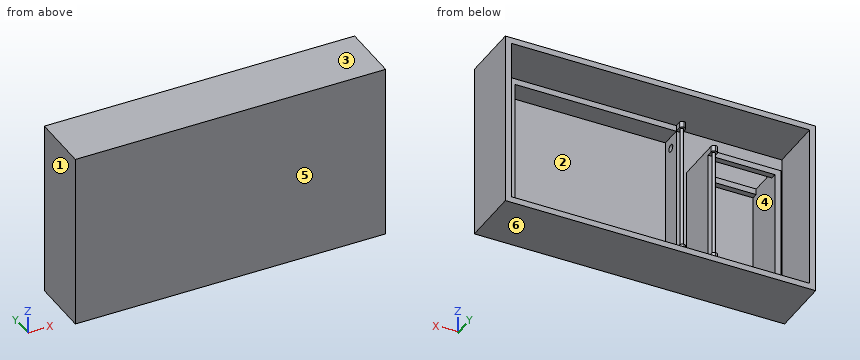
```python
from build123d import *

# Parameters (mm, degrees)
SKETCH1_W              = 127
SKETCH1_H              = 69.85
BASE_DEPTH             = 2.54
SKETCH2_W              = 73.66
SKETCH2_H              = 58.42
SKETCH2_W_2            = 68.58
SKETCH2_H_2            = 53.34
PCB_HOLDER_DEPTH       = 8.89
SKETCH1_3_W            = 132.08
SKETCH1_3_H            = 74.93
SKETCH1_3_W_2          = 127
SKETCH1_3_H_2          = 69.85
BOSS_EXTRUDE5_DEPTH    = 25.4
BOSS_EXTRUDE6_DEPTH    = 17.78
SKETCH7_W              = 25.908
SKETCH7_H              = 12.7
BATTERY_GAP_DEPTH      = 2.54
SKETCH4_R              = 1.5875
WIRE_GAP_DEPTH         = 2.54
SKETCH8_W              = 2.54
SKETCH8_H              = 2.54
PCB_HOLDER_HINGE_DEPTH = 3.81
FILLET4_R              = 1.27
SKETCH13_R             = 0.635
BOSS_EXTRUDE10_DEPTH   = 53.34
SKETCH14_W             = 2.54
SKETCH14_H             = 2.54
BOSS_EXTRUDE11_DEPTH   = 3.81
FILLET5_R              = 1.27
SKETCH15_R             = 0.635
BOSS_EXTRUDE13_DEPTH   = 46.228


with BuildPart() as part:
    # Sketch1 → Base (new body)
    with BuildSketch(Plane(origin=(0, 0, 0), x_dir=(1, 0, 0), z_dir=(0, 1, 0))):
        Rectangle(SKETCH1_W, SKETCH1_H)
    extrude(amount=BASE_DEPTH)

    # Sketch2 → PCB-Holder (add)
    with BuildSketch(Plane(origin=(0, 2.54, 0), x_dir=(1, 0, 0), z_dir=(0, 1, 0))):
        with Locations((20.32, -0.635)):
            Rectangle(SKETCH2_W, SKETCH2_H)
        with Locations((20.32, -0.635)):
            Rectangle(SKETCH2_W_2, SKETCH2_H_2, mode=Mode.SUBTRACT)
    extrude(amount=PCB_HOLDER_DEPTH)

    # Sketch1<3> → Boss-Extrude5 (add)
    with BuildSketch(Plane(origin=(0, 0, 0), x_dir=(1, 0, 0), z_dir=(0, 1, 0))):
        Rectangle(SKETCH1_3_W, SKETCH1_3_H)
        Rectangle(SKETCH1_3_W_2, SKETCH1_3_H_2, mode=Mode.SUBTRACT)
    extrude(amount=BOSS_EXTRUDE5_DEPTH)

    # Sketch6 → Boss-Extrude6 (add)
    with BuildSketch(Plane(origin=(0, 2.54, 0), x_dir=(1, 0, 0), z_dir=(0, 1, 0))):
        Polygon((-51.308, -13.843), (-51.308, 34.925), (-53.848, 34.925), (-53.848, -16.383), (-22.86, -16.383), (-22.86, 34.925), (-25.4, 34.925), (-25.4, -13.843), align=None)
    extrude(amount=BOSS_EXTRUDE6_DEPTH)

    # Sketch7 → Battery-Gap (cut)
    with BuildSketch(Plane.XY.offset(16.383)):
        with Locations((-38.354, 11.43)):
            Rectangle(SKETCH7_W, SKETCH7_H)
    extrude(amount=-BATTERY_GAP_DEPTH, mode=Mode.SUBTRACT)

    # Sketch4 → Wire-Gap (cut)
    with BuildSketch(Plane.ZY.offset(16.51)):
        with Locations((22.225, 6.985)):
            Circle(SKETCH4_R)
    extrude(amount=-WIRE_GAP_DEPTH, mode=Mode.SUBTRACT)

    # Sketch8 → PCB-Holder-Hinge (add)
    with BuildSketch(Plane(origin=(0, 11.43, 0), x_dir=(1, 0, 0), z_dir=(0, 1, 0))):
        with Locations((-15.24, -28.575)):
            Rectangle(SKETCH8_W, SKETCH8_H)
        with Locations((-15.24, 27.305)):
            Rectangle(SKETCH8_W, SKETCH8_H)
    extrude(amount=PCB_HOLDER_HINGE_DEPTH)

    # Fillet4
    fillet4_edges = [part.edges().sort_by_distance(p)[0] for p in [
        (-16.51, 15.24, -27.305),
        (-13.97, 15.24, -27.305),
        (-13.97, 15.24, 28.575),
        (-16.51, 15.24, 28.575),
    ]]
    fillet(fillet4_edges, radius=FILLET4_R - 0.0001)  # a hair under: the kernel refuses the full size

    # Sketch13 → Boss-Extrude10 (add)
    with BuildSketch(Plane.XY.offset(-26.035)):
        with Locations(Location((-15.24, 13.589, 0), (0, 0, 180))):
            Circle(SKETCH13_R)
    extrude(amount=BOSS_EXTRUDE10_DEPTH)

    # Sketch14 → Boss-Extrude11 (add)
    with BuildSketch(Plane(origin=(0, 20.32, 0), x_dir=(1, 0, 0), z_dir=(0, 1, 0))):
        with Locations((-24.13, -15.113)):
            Rectangle(SKETCH14_W, SKETCH14_H)
        with Locations((-24.13, 33.655)):
            Rectangle(SKETCH14_W, SKETCH14_H)
    extrude(amount=BOSS_EXTRUDE11_DEPTH)

    # Fillet5
    fillet5_edges = [part.edges().sort_by_distance(p)[0] for p in [
        (-22.86, 24.13, -33.655),
        (-25.4, 24.13, -33.655),
        (-25.4, 24.13, 15.113),
        (-22.86, 24.13, 15.113),
    ]]
    fillet(fillet5_edges, radius=FILLET5_R - 0.0001)  # a hair under: the kernel refuses the full size

    # Sketch15 → Boss-Extrude13 (add)
    with BuildSketch(Plane.XY.offset(-32.385)):
        with Locations(Location((-24.13, 22.479, 0), (0, 0, 180))):
            Circle(SKETCH15_R)
    extrude(amount=BOSS_EXTRUDE13_DEPTH)


solid = part.part
```
Check sheet for the modelled part. Datum: model origin and axes. Units: mm. Face numbers are marked on the shaded views. A direction names the side the tool comes from. Coordinates: 2 decimals unless noted, no trailing zeros. Loops run counter-clockwise (first coordinate to the right, second up) from the corner with the lowest first, then second, coordinate; pieces in that order, holes last. Notation, with made-up numbers: M -19,56.25 L -5,56.25 A29 cw -5,78.25 Z; hole C -5,9.5 d6. An arc over 180 degrees is marked long. Answer as a JSON object with one key per item and string values.
1. Access from +Z, -Z, +X, -X, +Y, -Y to the whole of each face (thin tool, end or side, straight path). Record for the marked faces 1 and 2.
Outcome:
{"face 1": "+Z, -Z, -X, +Y, -Y", "face 2": "+Y"}
2. Release check for a two-part mould opening along Z. For the marked faces 3, 4, 5 and 6 record: pulls with the +Z half, pulls with the -Z half, needs draft (parallel to the pull), parting line crosses it, or undercut.
Outcome:
{"face 3": "pulls with the +Z half", "face 4": "undercut", "face 5": "needs draft", "face 6": "pulls with the -Z half"}
3. Sectioned sample at D-D on x = -20. Record the cut outline in (y, z) (3 decimals), and give its area (3 significant figures).
Outcome:
{"outline": "M 0,-37.465 L 25.4,-37.465 L 25.4,-34.925 L 2.54,-34.925 L 2.54,34.925 L 25.4,34.925 L 25.4,37.465 L 0,37.465 Z", "area": "306 mm²"}
4. Sectioned sample at A-A on x = -40.5. Record the cut outline in (y, z) (3 decimals).
Outcome:
{"outline": "M 0,-37.465 L 25.4,-37.465 L 25.4,-34.925 L 2.54,-34.925 L 2.54,13.843 L 5.08,13.843 L 5.08,16.383 L 2.54,16.383 L 2.54,34.925 L 25.4,34.925 L 25.4,37.465 L 0,37.465 Z; M 17.78,13.843 L 20.32,13.843 L 20.32,16.383 L 17.78,16.383 Z"}
5. Sectioned sample at C-C on z = 32. Record the cut outline in (x, y).
Outcome:
{"outline": "M -66.04,0 L 66.04,0 L 66.04,25.4 L 63.5,25.4 L 63.5,2.54 L -63.5,2.54 L -63.5,25.4 L -66.04,25.4 Z"}
6. Scan lines: L1, parallel to Z at x = 30, y = 7.5 (3 decimals); L2, parallel to X at y = 11.5, z = -15.5; L3, parallel to X at y = 3, z = 25. Record each from-to range of solid material in increasing order. Write a range as from..to.
Outcome:
{"L1": "-37.465..-34.925, -28.575..-26.035, 27.305..29.845, 34.925..37.465", "L2": "-66.04..-63.5, -53.85..-51.31, -25.4..-22.86, 63.5..66.04", "L3": "-66.04..-63.5, -16.51..-13.97, 54.61..57.15, 63.5..66.04"}
7. Sectioned sample at B-B on z = 3. Record the cut outline in (x, y) (3 decimals), and give its area (3 significant figures).
Outcome:
{"outline": "M -66.04,0 L 66.04,0 L 66.04,25.4 L 63.5,25.4 L 63.5,2.54 L 57.15,2.54 L 57.15,11.43 L 54.61,11.43 L 54.61,2.54 L -13.97,2.54 L -13.97,11.43 L -16.51,11.43 L -16.51,2.54 L -22.86,2.54 L -22.86,20.32 L -25.4,20.32 L -25.4,2.54 L -51.308,2.54 L -51.308,20.32 L -53.848,20.32 L -53.848,2.54 L -63.5,2.54 L -63.5,25.4 L -66.04,25.4 Z; C -24.13,22.479 d1.27; C -15.24,13.589 d1.27", "area": "590 mm²"}
8. Depth check by flat-ended pin: P1, Ø12, axis at x = 44.5, z = -28, coming from the +Y side; P2, Ø2, axis at x = 40.5, z = 2, coming from the +Y side. Enter the tip coordinate at first touch or a pass-through.
Outcome:
{"P1": "y = 11.43", "P2": "y = 2.54"}
